Autodesk Inventor part; units mm, degrees
ref_plane "Work Plane1" through (0, 0, 2) normal (0, 0, -1) x (-1, 0, 0)
ref_plane "YZ Plane" through (0, 0, 0) normal (1, 0, 0) x (0, 1, 0)
ref_plane "XZ Plane" through (0, 0, 0) normal (0, 1, 0) x (-1, 0, 0)
sketch "Sketch1" plane through (0, 0, 0) normal (0, 0, 1) x (1, 0, 0)
  arc A0 (13.5417, 29.5444) -> (13.5417, -29.5444) centre (0, 0) ccw
  arc A1 (38.3333, -18.1812) -> (38.3333, 18.1812) centre (30, 0) ccw
  line L0 (0, 0) -> (30, 0)
  line L1 (13.5417, 29.5444) -> (38.3333, 18.1812)
  line L2 (13.5417, -29.5444) -> (38.3333, -18.1812)
  dimension "d0" = 65
  dimension "d1" = 40
  dimension "d2" = 30
extrude "Extrusion1" add sketch "Sketch1" along normal blind 3
chamfer "Chamfer1" distance 5 distance2 2 4 edges at (50, 0, 3) (25.9375, 23.8628, 3) (-32.5, 0, 3) (25.9375, -23.8628, 3) measured on face at (-1.7306, 1.2719, 3)
sketch "Sketch2" plane through (0, 0, 0) normal (0, 0, -1) x (-1, 0, 0)
  line L0 (-13.5417, -29.5444) -> (-38.3333, -18.1812) construction
  arc A0 (-13.5417, -29.5444) -> (-13.5417, 29.5444) centre (0, 0) ccw construction
  line L1 (-38.3333, 18.1812) -> (-13.5417, 29.5444) construction
  arc A1 (-38.3333, 18.1812) -> (-38.3333, -18.1812) centre (-30, 0) ccw construction
  arc A2 (-10.625, -23.181) -> (-10.625, 23.181) centre (0, 0) ccw construction
  line L2 (-10.625, -23.181) -> (-35.4167, -11.8178) construction
  arc A3 (-35.4167, 11.8178) -> (-35.4167, -11.8178) centre (-30, 0) ccw construction
  line L3 (-35.4167, 11.8178) -> (-10.625, 23.181) construction
  line L4 (0, 0) -> (12.75, 22.0836) construction
  line L5 (0, 0) -> (12.75, -22.0836) construction
  circle A4 centre (-30.0011, 14.3) radius 0.65
  circle A5 centre (-30.0011, -14.3) radius 0.65
  circle A6 centre (12.75, -22.0836) radius 0.65
  circle A7 centre (12.75, 22.0836) radius 0.65
  line L6 (0, 0) -> (25.5, 0) construction
  dimension "d8" = 7
  dimension "d11" = 1.3
  dimension "d12" = 1.3
  dimension "d13" = 1.3
  dimension "d14" = 1.3
  dimension "d25" = 13
  dimension "d26" = 14.3
  dimension "d27" = 14.3
  dimension "d28" = 120
  dimension "d29" = 60
extrude "Extrusion2" cut sketch "Sketch2" against normal blind 10
ref_plane "Work Plane1" through (0, 0, 2) normal (0, 0, -1) x (-1, 0, 0)
sketch "Sketch3" plane through (0, 0, 2) normal (0, 0, -1) x (-1, 0, 0)
  circle A0 centre (12.75, -22.0836) radius 0.65
  circle A1 centre (-30.0011, -14.3) radius 0.65
  circle A2 centre (12.75, 22.0836) radius 0.65
  circle A3 centre (-30.0011, 14.3) radius 0.65
  line L0 (-13.5417, -29.5444) -> (-38.3333, -18.1812)
  arc A4 (-13.5417, -29.5444) -> (-13.5417, 29.5444) centre (0, 0) ccw
  line L1 (-38.3333, 18.1812) -> (-13.5417, 29.5444)
  arc A5 (-38.3333, 18.1812) -> (-38.3333, -18.1812) centre (-30, 0) ccw
  circle A6 centre (-30.0011, 14.3) radius 1.65
  circle A7 centre (-30.0011, -14.3) radius 1.65
  circle A8 centre (12.75, -22.0836) radius 1.65
  circle A9 centre (12.75, 22.0836) radius 1.65
  dimension "d18" = 3.3
  dimension "d19" = 3.3
  dimension "d20" = 3.3
  dimension "d21" = 3.3
extrude "Extrusion3" cut sketch "Sketch3" against normal blind 10 contours A0 | A1 | A2 | A3 | A6 | A7 | A8 | A9
properties part number "Wirst_2R_cover"
Work out the finished part from the listing and answer in its coordinate system (mm). A direction names the side the tool comes from. Round coordinates to 2 decimals unless told otherwise and drop trailing zeros. Write each loop counter-clockwise with the first axis right and the second up, starting at its lowest first coordinate (ties: lowest second). Pieces come first, ordered by that corner, then holes. Notation, with made-up numbers: (10.25, -8) -> (35.25, -8) arc R25 ccw to (35.25, 28) -> close; hole circle Ø10 at (33.5, 29.25). An arc over 180 degrees is marked (long way). Write each question's results on one line, items separated by ' | '.
Item 1: A cutting plane is placed at A-A, the plane y = 0. Determine the outline of the cut face in (x, z).
Result set:
outline: (-32.5, 0) -> (50, 0) -> (50, 1) -> (45, 3) -> (-27.5, 3) -> (-32.5, 1) -> close
Item 2: The mould has two halves that part along Y. Classify faces 3 (the face through (31.31, -15.304, 2.493)), 4 (the face through (25.764, -23.942, 0.493)), 5 (the face through (24.737, 21.702, 1.986)): +Y half, -Y half, draft (parallel to the pull), parting line (faces both ways), or undercut.
Result set:
face 3: undercut | face 4: -Y half | face 5: +Y half
Item 3: A cutting plane is placed at B-B, the plane x = 0. Determine the outline of the cut face in (y, z).
Result set:
outline: (-32.5, 0) -> (32.5, 0) -> (32.5, 1) -> (27.5, 3) -> (-27.5, 3) -> (-32.5, 1) -> close
Item 4: Find the intervals of material crossed by line 1 along Y through (x, z) = (-12.75, 0.65); line 2 along Y through (x, z) = (36.5, 0.45); line 3 along X through (y, z) = (-2, 0.95), in increasing order. Write a range as [from, to].
Result set:
line 1: [-29.89, -22.73], [-21.43, 21.43], [22.73, 29.89] | line 2: [-19.02, 19.02] | line 3: [-32.44, 49.9]
Item 5: Which of the six approach directions +Z, -Z, +X, -X, +Y, -Y give full straight-line access (tool end or side, diameter ignored) to faces 1 (the face through (31.217, 15.415, 2.493)), 2 (the face through (8, 0, 3))?
Result set:
face 1: +Z | face 2: +Z, +X, -X, +Y, -Y
Item 6: Flat-ended cylindrical pins translate along their axes: P1, Ø1, axis at x = -11, z = 1, coming from the +Y side; P2, Ø1.6, axis at x = -12.5, y = -21.5, coming from the +Z side; P3, Ø1.2, axis at x = 30, y = -14.3, coming from the -Z side. Find the tip coordinate at first contact, or state that the pin passes through.
Result set:
P1: y = 30.76 | P2: z = 2 | P3: through
